Input: part model. Units: mm. Frame: model coordinates. Face numbers are marked on the shaded views. A direction names the side the tool comes from. Coordinates: 2 decimals unless noted, no trailing zeros. Loops run counter-clockwise (first coordinate to the right, second up) from the corner with the lowest first, then second, coordinate; pieces in that order, holes last. Notation, with made-up numbers: (89, 73) -> (104, 73) arc R27 ccw to (104, 98) -> close; hole circle Ø11 at (30.25, -31.75). An arc over 180 degrees is marked (long way). Answer as a JSON object with one key per item and string values.
from build123d import *

# Parameters (mm, degrees)
BOSS_EXTRU_1_DEPTH      = 4
BOSS_EXTRU_2_DEPTH      = 20
ESQUISSE3_R             = 3
ENL_V_MAT_EXTRU_1_DEPTH = 25
ESQUISSE4_R             = 3
ENL_V_MAT_EXTRU_2_DEPTH = 25
ESQUISSE5_R             = 2.25
ENL_V_MAT_EXTRU_3_DEPTH = 5
CONG_1_R                = 6


with BuildPart() as part:
    # Esquisse1 → Boss.-Extru.1 (new body)
    with BuildSketch(Plane.XY):
        Polygon((-20, 60), (-20, 40), (-40, 40), (-40, 0), (0, 0), (0, 20), (20, 20), (20, 60), align=None)
    extrude(amount=BOSS_EXTRU_1_DEPTH)

    # Esquisse2 → Boss.-Extru.2 (add)
    with BuildSketch(Plane.XY.offset(4)):
        Polygon((20, 20), (20, 24), (-4, 24), (-4, 0), (0, 0), (0, 20), align=None)
    extrude(amount=BOSS_EXTRU_2_DEPTH)

    # Esquisse3 → Enlèv. mat.-Extru.1 (cut, through all)
    with BuildSketch(Plane.ZY.offset(4)):
        with Locations(Location((14, 10, 0), (0, 0, 270))):  # turned: the seam where the file's is
            Circle(ESQUISSE3_R)
    extrude(amount=-ENL_V_MAT_EXTRU_1_DEPTH, mode=Mode.SUBTRACT)

    # Esquisse4 → Enlèv. mat.-Extru.2 (cut, through all)
    with BuildSketch(Plane(origin=(0, 24, 0), x_dir=(1, 0, 0), z_dir=(0, 1, 0))):
        with Locations(Location((10, -14, 0), (0, 0, 180))):  # turned: the seam where the file's is
            Circle(ESQUISSE4_R)
    extrude(amount=-ENL_V_MAT_EXTRU_2_DEPTH, mode=Mode.SUBTRACT)

    # Esquisse5 → Enlèv. mat.-Extru.3 (cut, through all)
    with BuildSketch(Plane.XY.offset(4)):
        with Locations((10, 50)):
            Circle(ESQUISSE5_R)
        with Locations((-10, 50)):
            Circle(ESQUISSE5_R)
        with Locations((-30, 30)):
            Circle(ESQUISSE5_R)
        with Locations((-30, 10)):
            Circle(ESQUISSE5_R)
    extrude(amount=-ENL_V_MAT_EXTRU_3_DEPTH, mode=Mode.SUBTRACT)

    # Congé1
    cong_1_edges = [part.edges().sort_by_distance(p)[0] for p in [
        (-40, 40, 2),
        (-20, 40, 2),
        (-20, 60, 2),
    ]]
    fillet(cong_1_edges, radius=CONG_1_R)


solid = part.part
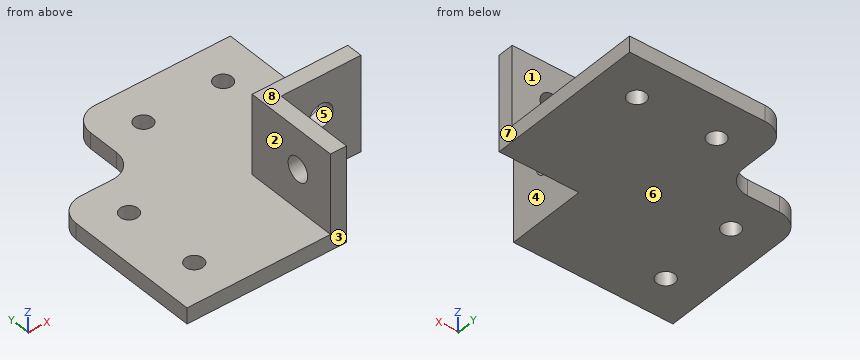
1. Mould query, pull axis Z, two halves, no side actions, for the marked faces 5, 6, 7 and 8. Classes: pulls with the +Z half, pulls with the -Z half, needs draft (parallel to the pull), parting line crosses it, or undercut.
Reply:
{"face 5": "undercut", "face 6": "pulls with the -Z half", "face 7": "needs draft", "face 8": "pulls with the +Z half"}
2. Section query B-B (x = -10). Return loops of the section in (y, z), plus the area to 3 significant figures.
Reply:
{"outline": "(0, 0) -> (47.75, 0) -> (47.75, 4) -> (0, 4) -> close; (52.25, 0) -> (60, 0) -> (60, 4) -> (52.25, 4) -> close", "area": "222 mm2"}
3. Section query C-C (y = 30). Return loops of the section in (x, z).
Reply:
{"outline": "(-40, 0) -> (-32.25, 0) -> (-32.25, 4) -> (-40, 4) -> close; (-27.75, 0) -> (20, 0) -> (20, 4) -> (-27.75, 4) -> close"}
4. Section query A-A (z = 14). Return loops of the section in (x, y).
Reply:
{"outline": "(-4, 0) -> (0, 0) -> (0, 7) -> (-4, 7) -> close; (-4, 13) -> (0, 13) -> (0, 20) -> (7, 20) -> (7, 24) -> (-4, 24) -> close; (13, 20) -> (20, 20) -> (20, 24) -> (13, 24) -> close"}
5. Line query: line 1 along Y through (x, z) = (-30, 1.35); line 2 along Z through (x, y) = (-1.3, 10); line 3 along Y through (x, z) = (-10, 1). Output: solid intervals per line, ascending.
Reply:
{"line 1": "y = 0 to 7.75, 12.25 to 27.75, 32.25 to 40", "line 2": "z = 0 to 11, 17 to 24", "line 3": "y = 0 to 47.75, 52.25 to 60"}
6. Access query for the marked faces 1, 2, 3 and 4. Directions: +Z, -Z, +X, -X, +Y, -Y. A direction counts if a zero-diameter tool reaches every point of the face in a straight line with its end or side. Return the directions, or none.
Reply:
{"face 1": "+Z, +X, -X, +Y", "face 2": "+Z, -X, +Y, -Y", "face 3": "+Z, -Z, +X, -X, -Y", "face 4": "+Z, -Z, +X, -Y"}
7. Pin query (flat end, axial travel): P1, Ø9.5, axis at x = 10, z = 14, coming from the -Y side; P2, Ø6, axis at y = 9.5, z = 14, coming from the -X side; P3, Ø2, axis at y = 49, z = 1, coming from the -X side. Return the tip coordinate at first contact, or that it passes through.
Reply:
{"P1": "stops at y = 20", "P2": "stops at x = -4", "P3": "stops at x = -20"}
8. Section query D-D (x = 10). Return loops of the section in (y, z).
Reply:
{"outline": "(20, 0) -> (47.75, 0) -> (47.75, 4) -> (24, 4) -> (24, 11) -> (20, 11) -> close; (20, 17) -> (24, 17) -> (24, 24) -> (20, 24) -> close; (52.25, 0) -> (60, 0) -> (60, 4) -> (52.25, 4) -> close"}
